Geometry check sheet. Reference: drawing and pictorial views, mm from the part's lowest x, y, z. Round coordinates to 2 decimals unless told otherwise and drop trailing zeros. Order: outer loops, then holes, each group sorted by start corner. A loop starts at its lowest first (then second) coordinate and runs counter-clockwise, first axis right, second up.
(1) Mould release check, pull along Y, two halves, no side actions. Record for the marked faces 1 and 2: released by +Y, released by -Y, zero draft, split by the parting line, or undercut.
(2) Sectioned sample at B-B, the plane y = 25.5. Enter the section's corners in (x, z).
(3) Depth check by flat-ended pin: pin 1 (5.5 mm diameter, centred on x = 27.46, y = 27.54, fed in from -Z). Enter the tip coordinate at first touch or a pass-through.
(4) Sectioned sample at C-C, the plane x = 27. Enter the section's corners in (y, z).
(5) Thickness scan on probe 1 along X at (y, z) = (28.5, 0.25); probe 2 along Y at (x, z) = (50.5, 1.5); probe 3 along X at (y, z) = (27, 0.65). Record the ranges inside material, lowest first.
(6) Sectioned sample at A-A, the plane z = 0.45. Enter the section's corners in (x, y), and give its area (3 significant figures).
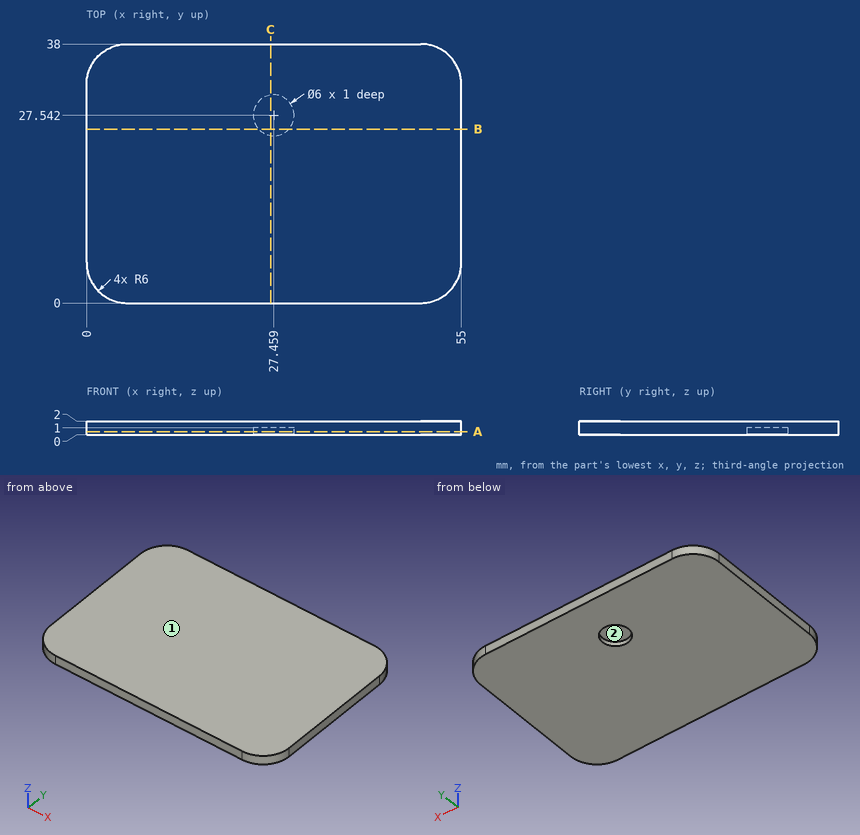
Derived:
1. face 1: zero draft
1. face 2: undercut
2. outline: (0, 0) - (25.26, 0) - (25.26, 1) - (29.66, 1) - (29.66, 0) - (55, 0) - (55, 2) - (0, 2) - close
3. pin 1: stops at z = 1
4. outline: (0, 0) - (24.58, 0) - (24.58, 1) - (30.51, 1) - (30.51, 0) - (38, 0) - (38, 2) - (0, 2) - close
5. probe 1: x = 0 to 24.62, 30.3 to 55
5. probe 2: y = 0.19 to 37.81
5. probe 3: x = 0 to 24.51, 30.41 to 55
6. outline: (0, 6) arc R6 ccw to (6, 0) - (49, 0) arc R6 ccw to (55, 6) - (55, 32) arc R6 ccw to (49, 38) - (6, 38) arc R6 ccw to (0, 32) - close; hole circle Ø6 at (27.46, 27.54)
6. area: 2,030 mm2
